from build123d import *

# Parameters (mm, degrees)
SALIENTE_EXTRUIR2_DEPTH = 5


with BuildPart() as part:
    # Croquis1 → Saliente-Extruir2 (new body)
    with BuildSketch(Plane(origin=(0, 0, 0), x_dir=(1, 0, 0), z_dir=(0, 1, 0))):
        with BuildLine():
            Line((0, 0), (13, 0))
            Line((13, 0), (13, 7.6962052))
            ThreePointArc((13, 7.6962052), (15.928932188, 14.767273012), (23, 17.6962052))
            Line((23, 17.6962052), (53, 17.6962052))
            ThreePointArc((53, 17.6962052), (60.071067812, 14.767273012), (63, 7.6962052))
            Line((63, 7.6962052), (63, 0))
            Line((63, 0), (76, 0))
            Line((76, 0), (76, 13.554999328))
            ThreePointArc((76, 13.554999328), (73.071067812, 20.62606714), (66, 23.554999328))
            Line((66, 23.554999328), (10, 23.554999328))
            ThreePointArc((10, 23.554999328), (2.928932188, 20.62606714), (0, 13.554999328))
            Line((0, 13.554999328), (0, 0))
        make_face()
    extrude(amount=SALIENTE_EXTRUIR2_DEPTH)


solid = part.part
Geometry: final body of the model. Coordinates: model frame, mm. A direction names the side the tool comes from. Give positions to 0.01 mm unless a question says otherwise; leave off trailing zeros. Write each loop counter-clockwise with the first axis right and the second up, starting at its lowest first coordinate (ties: lowest second). Pieces come first, ordered by that corner, then holes.
(1) Cut plane A-A, the plane z = -6.25. Return loops of the section in (x, y).
(2) Mould query, pull axis X, two halves, no side actions, for faces 3 (the flat face through (76, 2, -7)), 4 (the flat face through (38, 2, -17.696)), 5 (the flat face through (13, 2, -4)), 6 (the flat face through (6, 2, 0)). Classes: released by +X, released by -X, zero draft, split by the parting line, or undercut.
(3) Ray query, line 1 (X direction, y = 4.4, z = -4); line 2 (Z direction, x = 39.5, y = 0.7) (3 decimals); line 3 (X direction, y = 3.5, z = -11). Return the intervals inside material, ascending.
(4) Access query for faces 1 (the flat face through (38, 2, -23.555)), 2 (the cylindrical face through (59.993, 2.465, -14.845)). Directions: +Z, -Z, +X, -X, +Y, -Y. A direction counts if a zero-diameter tool reaches every point of the face in a straight line with its end or side. Return the directions, or none.
(5) Cut plane C-C, the plane x = 47. Return loops of the section in (y, z) (3 decimals), then the cut area to 3 significant figures.
(6) Cut plane B-B, the plane y = 0.75. Return loops of the section in (x, z) (3 decimals), then the cut area to 3 significant figures.
(7) Cut plane D-D, the plane z = -15.5. Return loops of the section in (x, y), then the cut area to 3 significant figures.
(8) First-contact query: P1, Ø1.5, axis at y = 4, z = -19.5, coming from the -X side. Flat tip, straight axial feed; report the tip coordinate or a pass-through.
Values follow:
1. outline: (0, 0) - (13, 0) - (13, 5) - (0, 5) - close; (63, 0) - (76, 0) - (76, 5) - (63, 5) - close
2. face 3: released by +X
2. face 4: undercut
2. face 5: undercut
2. face 6: zero draft
3. line 1: x = 0 to 13, 63 to 76
3. line 2: z = -23.555 to -17.696
3. line 3: x = 0 to 13.56, 62.44 to 76
4. face 1: -Z, +X, -X, +Y, -Y
4. face 2: +Z, +Y, -Y
5. outline: (0, -23.555) - (5, -23.555) - (5, -17.696) - (0, -17.696) - close
5. area: 29.3 mm2
6. outline: (0, -13.555) arc R10 ccw to (10, -23.555) - (66, -23.555) arc R10 ccw to (76, -13.555) - (76, 0) - (63, 0) - (63, -7.696) arc R10 cw to (53, -17.696) - (23, -17.696) arc R10 cw to (13, -7.696) - (13, 0) - (0, 0) - close
6. area: 905 mm2
7. outline: (0.19, 0) - (16.75, 0) - (16.75, 5) - (0.19, 5) - close; (59.25, 0) - (75.81, 0) - (75.81, 5) - (59.25, 5) - close
7. area: 166 mm2
8. P1: stops at x = 1.46
